The model under review builds one solid part; all positions refer to its coordinate system, in mm. A direction names the side the tool comes from. Coordinates: 2 decimals unless noted, no trailing zeros. Loops run counter-clockwise (first coordinate to the right, second up) from the corner with the lowest first, then second, coordinate; pieces in that order, holes last. Notation, with made-up numbers: M 27.25,-38 L 83.25,-38 A26 ccw 83.25,-2 Z; hole C 56.5,18 d11. An arc over 180 degrees is marked long. Use one line per item in the form item = value.
```python
from build123d import *

# Parameters (mm, degrees)
SKETCH1_R      = 4
EXTRUDE1_DEPTH = 13
FILLET5_R      = 5
SKETCH5_R      = 4
EXTRUDE5_DEPTH = 30
SKETCH6_R      = 4
EXTRUDE6_DEPTH = 30
SKETCH8_R      = 4
EXTRUDE7_DEPTH = 30


with BuildPart() as part:
    # Sketch1 → Extrude1 (new body)
    with BuildSketch(Plane(origin=(0, 0, 0), x_dir=(1, 0, 0), z_dir=(0, 1, 0))):
        Polygon((0, -15), (-15, 0), (-42, 0), (-42, 30), (-2.573593129, 30), (30, -2.573593129), (30, -42), (0, -42), align=None)
        with Locations((-8.786796564, 15)):
            Circle(SKETCH1_R, mode=Mode.SUBTRACT)
        with Locations((15, -8.786796564)):
            Circle(SKETCH1_R, mode=Mode.SUBTRACT)
    extrude(amount=EXTRUDE1_DEPTH)

    # Fillet5
    fillet5_edges = [part.edges().sort_by_distance(p)[0] for p in [
        (-42, 6.5, 0),
        (-42, 6.5, -30),
        (-2.573593129, 6.5, -30),
        (30, 6.5, 2.573593129),
        (30, 6.5, 42),
        (0, 6.5, 42),
        (0, 6.5, 15),
        (-15, 6.5, 0),
    ]]
    fillet(fillet5_edges, radius=FILLET5_R)

    # Sketch5 → Extrude5 (cut)
    with BuildSketch(Plane(origin=(-7.5, 0, 7.5), x_dir=(0.707106781, 0, 0.707106781), z_dir=(-0.707106781, 0, 0.707106781))):
        with Locations((0, 6.5)):
            Circle(SKETCH5_R)
    extrude(amount=-EXTRUDE5_DEPTH, mode=Mode.SUBTRACT)

    # Sketch6 → Extrude6 (cut)
    with BuildSketch(Plane.XY):
        with Locations((-28, 6.5)):
            Circle(SKETCH6_R)
    extrude(amount=-EXTRUDE6_DEPTH, mode=Mode.SUBTRACT)

    # Sketch8 → Extrude7 (cut)
    with BuildSketch(Plane.ZY):
        with Locations((28, 6.5)):
            Circle(SKETCH8_R)
    extrude(amount=-EXTRUDE7_DEPTH, mode=Mode.SUBTRACT)


solid = part.part
```
1. Insertion check: P1, Ø6, axis at y = 9, z = 22, coming from the -X side; P2, Ø5, axis at x = -28, y = 6.5, coming from the +Z side; P3, Ø6, axis at x = 4.5, y = 1.5, coming from the -Z side; P4, Ø4, axis at x = -32.5, y = 4.5, coming from the +Z side. Each pin has a flat end and moves straight along its axis. Give the tip position at first contact, or say it passes through.
Response values:
P1 = 0
P2 = through
P3 = -25.93
P4 = 0
2. Machinability: for faces 5 (the face through (29.63, 6.59, 2.76)), 6 (the face through (0, 3.5, 25)), which of the approach directions +Z, -Z, +X, -X, +Y, -Y give a long, thin tool a straight path to every point of the face, cutting with its end or side? Answer none if there is none.
Response values:
face_5 = -Z, +X, +Y, -Y
face_6 = +Z, -X, +Y, -Y
3. The part is to be moulded in two halves that separate along X. For faces 1 (the face through (-4.7, 7.9, 10.3)), 2 (the face through (-21, 6, -30)), 3 (the face through (28, 7, 41)), 4 (the face through (-31.2, 4.1, -14.8)), say which applies: pulls with the +X half, pulls with the -X half, needs draft (parallel to the pull), parting line crosses it, or undercut.
Response values:
face_1 = pulls with the -X half
face_2 = needs draft
face_3 = pulls with the +X half
face_4 = undercut
4. Add section A-A (y = 5.5). Count the separate pieces of the cut face and the enclosed holes in it, then the cut area to 3 significant figures.
Response values:
separate_pieces = 4
enclosed_holes = 2
area = 2,180 mm^2
5. Add section B-B (z = 28). State the section outline as (x, y) points, then the cut area to 3 significant figures.
Response values:
outline = M 0,0 L 30,0 L 30,2.5 L 0,2.5 Z; M 0,10.5 L 30,10.5 L 30,13 L 0,13 Z
area = 150 mm^2
6. Add section C-C (y = 11.5). State the section outline as (x, z) points.
Response values:
outline = M -42,-25 A5 ccw -37,-30 L -4.64,-30 A5 ccw -1.11,-28.54 L 28.54,1.11 A5 ccw 30,4.64 L 30,37 A5 ccw 25,42 L 5,42 A5 ccw 0,37 L 0,17.07 A5 cw -1.46,13.54 L -13.54,1.46 A5 cw -17.07,0 L -37,0 A5 ccw -42,-5 Z; hole C -8.79,-15 d8; hole C 15,8.79 d8
7. Wall thickness on line 1 along X through (y, z) = (5.25, -3); line 2 along Z through (x, y) = (9, 3.5); line 3 along Z through (x, y) = (15, 9.5): over which ranges is each line inside the solid? List them lowest first. Write a range as from..to.
Response values:
line_1 = -41.58..-31.8, -24.2..-2.37, 8.37..24.43
line_2 = -18.43..-12.74, -5.26..25.35, 30.65..42
line_3 = -11.26..4.79, 12.79..25.35, 30.65..42
